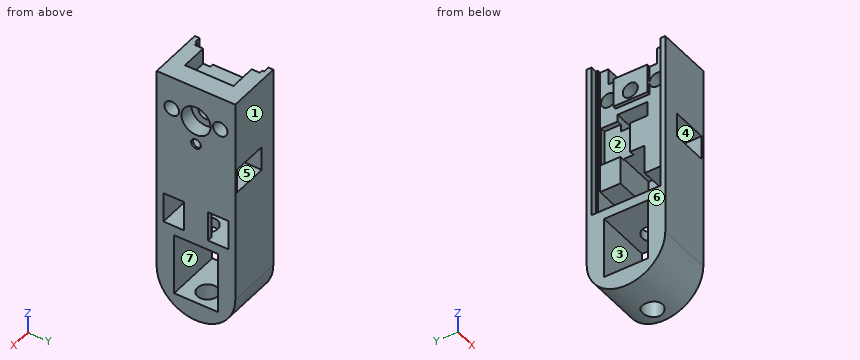
```python
from build123d import *

# Parameters (mm, degrees)
SKETCH_W         = 4.2
SKETCH_H         = 6.2
EXTRUDE_DEPTH    = 11.5
SKETCH001_W      = 14.2
SKETCH001_H      = 32.3
SKETCH001_R      = 1.55
EXTRUDE001_DEPTH = 1.3
SKETCH003_W      = 10
SKETCH003_H      = 4.382065
EXTRUDE003_DEPTH = 7.5
SKETCH004_W      = 13.4
SKETCH004_H      = 32.3
SKETCH004_W_2    = 7
SKETCH004_H_2    = 6
EXTRUDE004_DEPTH = 2
SKETCH005_W      = 6
SKETCH005_H      = 8
EXTRUDE005_DEPTH = 3
SKETCH009_W      = 18
SKETCH009_H      = 5
EXTRUDE013_DEPTH = 7.5
SKETCH012_W      = 9
SKETCH012_H      = 12.7
EXTRUDE014_DEPTH = 11.5
SKETCH011_R      = 2.08
EXTRUDE012_DEPTH = 20
SKETCH002_W      = 5
SKETCH002_H      = 12.2
EXTRUDE011_DEPTH = 10.5
EXTRUDE015_DEPTH = 3
SKETCH014_R      = 1
EXTRUDE016_DEPTH = 12
SKETCH015_R      = 1.5
EXTRUDE017_DEPTH = 11.5
SKETCH016_R      = 3
EXTRUDE018_DEPTH = 3
SKETCH010_R      = 1.55
EXTRUDE010_DEPTH = 12
EXTRUDE006_DEPTH = 11.5


with BuildPart() as extrude_body:
    # Sketch → Extrude (new body)
    with BuildSketch(Plane.YZ):
        with Locations((4.6, 3.1)):
            Rectangle(SKETCH_W, SKETCH_H)
    extrude(amount=EXTRUDE_DEPTH)


with BuildPart() as extrude001:
    # Sketch001 → Extrude001 (new body)
    with BuildSketch(Plane.YZ):
        with Locations((0, 16.15)):
            Rectangle(SKETCH001_W, SKETCH001_H)
        with Locations((0, 25)):
            Circle(SKETCH001_R, mode=Mode.SUBTRACT)
    extrude(amount=EXTRUDE001_DEPTH)


with BuildPart() as extrude003:
    # Sketch003 → Extrude003 (new body)
    with BuildSketch(Plane.YZ):
        with Locations((0, 31.191032)):
            Rectangle(SKETCH003_W, SKETCH003_H)
    extrude(amount=EXTRUDE003_DEPTH)


with BuildPart() as extrude004:
    # Sketch004 → Extrude004 (new body)
    with BuildSketch(Plane.YZ):
        with Locations((0, 16.15)):
            Rectangle(SKETCH004_W, SKETCH004_H)
        with Locations((0, 26)):
            Rectangle(SKETCH004_W_2, SKETCH004_H_2, mode=Mode.SUBTRACT)
    extrude(amount=EXTRUDE004_DEPTH)


with BuildPart() as extrude005:
    # Sketch005 → Extrude005 (new body)
    with BuildSketch(Plane.YZ):
        with Locations((3.5, 16)):
            Rectangle(SKETCH005_W, SKETCH005_H)
    extrude(amount=EXTRUDE005_DEPTH)


with BuildPart() as board:
    # Part__Mirroring: instance of Extrude body
    add(extrude_body.part.mirror(Plane(origin=(0, 0, 0), x_dir=(1, 0, 0), z_dir=(0, 1, 0))))

    # Fusion: union Extrude body, Extrude001, Extrude003, Extrude004, Extrude005
    add(extrude_body.part)
    add(extrude001.part)
    add(extrude003.part)
    add(extrude004.part)
    add(extrude005.part)


with BuildPart() as obj1:
    # Sketch009 → Extrude013 (new body)
    with BuildSketch(Plane.YZ):
        with Locations((0, 15.2)):
            Rectangle(SKETCH009_W, SKETCH009_H)
    extrude(amount=EXTRUDE013_DEPTH)


with BuildPart() as obj1_1:
    # Extrude013 placement: moved
    add(obj1.part.moved(Location((3.5, 0, 0))))


with BuildPart() as obj2:
    # Sketch012 → Extrude014 (new body)
    with BuildSketch(Plane.YZ):
        with Locations((0, -8.35)):
            Rectangle(SKETCH012_W, SKETCH012_H)
    extrude(amount=EXTRUDE014_DEPTH)


with BuildPart() as percageaxe:
    # Sketch011 → Extrude012 (new body)
    with BuildSketch(Plane.XY):
        with Locations((8, 0)):
            Circle(SKETCH011_R)
    extrude(amount=-EXTRUDE012_DEPTH)


with BuildPart() as obj3:
    # Sketch002 → Extrude011 (new body)
    with BuildSketch(Plane.YZ):
        with Locations((0, 6.1)):
            Rectangle(SKETCH002_W, SKETCH002_H)
    extrude(amount=EXTRUDE011_DEPTH)


with BuildPart() as obj4:
    # Sketch013 → Extrude015 (new body)
    with BuildSketch(Plane.XY):
        with BuildLine():
            ThreePointArc((6.780369, -2.85), (11.1, 0), (6.780369, 2.85))
            ThreePointArc((6.780369, 2.85), (6.183233, 3.036857), (5.560738, 3.1))
            Line((5.560738, 3.1), (0, 3.1))
            Line((0, -3.1), (0, 3.1))
            Line((5.560738, -3.1), (0, -3.1))
            ThreePointArc((5.560738, -3.1), (6.183233, -3.036857), (6.780369, -2.85))
        make_face()
    extrude(amount=EXTRUDE015_DEPTH)


with BuildPart() as obj4_1:
    # Extrude015 placement: moved
    add(obj4.part.moved(Location((0, 0, 18.5))))


with BuildPart() as obj5:
    # Sketch014 → Extrude016 (new body)
    with BuildSketch(Plane.YZ):
        Circle(SKETCH014_R)
    extrude(amount=EXTRUDE016_DEPTH)


with BuildPart() as obj5_1:
    # Extrude016 placement: moved
    add(obj5.part.moved(Location((0, 0, 20))))


with BuildPart() as obj6:
    # Sketch015 → Extrude017 (new body)
    with BuildSketch(Plane.YZ):
        with Locations((-5, 25.5)):
            Circle(SKETCH015_R)
        with Locations((5, 25.5)):
            Circle(SKETCH015_R)
    extrude(amount=EXTRUDE017_DEPTH)


with BuildPart() as obj7:
    # Sketch016 → Extrude018 (new body)
    with BuildSketch(Plane.YZ):
        with Locations((0, 25)):
            Circle(SKETCH016_R)
    extrude(amount=EXTRUDE018_DEPTH)


with BuildPart() as obj7_1:
    # Extrude018 placement: moved
    add(obj7.part.moved(Location((8.5, 0, 0))))


with BuildPart() as fusion002:
    # Sketch010 → Extrude010 (new body)
    with BuildSketch(Plane.YZ):
        with Locations((0, 25)):
            Circle(SKETCH010_R)
    extrude(amount=EXTRUDE010_DEPTH)

    # Fusion002: union obj1, obj2, PercageAxe, obj3, obj4, obj5, obj6, obj7
    add(obj1_1.part)
    add(obj2.part)
    add(percageaxe.part)
    add(obj3.part)
    add(obj4_1.part)
    add(obj5_1.part)
    add(obj6.part)
    add(obj7_1.part)


with BuildPart() as cut001:
    # Sketch006 → Extrude006 (new body)
    with BuildSketch(Plane.YZ):
        with BuildLine():
            Line((-8.1, 32.3), (8.1, 32.3))
            Line((8.1, -10.5), (8.1, 32.3))
            ThreePointArc((-8.1, -10.5), (0, -18.6), (8.1, -10.5))
            Line((-8.1, 32.3), (-8.1, -10.5))
        make_face()
    extrude(amount=EXTRUDE006_DEPTH)

    # Cut: cut Fusion002
    add(fusion002.part, mode=Mode.SUBTRACT)

    # Cut001: cut Board
    add(board.part, mode=Mode.SUBTRACT)


solid = cut001.part
```
Work out the finished part from the listing and answer in its coordinate system (mm). Face numbers are marked on the shaded views. A direction names the side the tool comes from. Round coordinates to 2 decimals unless told otherwise and drop trailing zeros. Loops run counter-clockwise (first coordinate to the right, second up) from the corner with the lowest first, then second, coordinate; pieces in that order, holes last. Notation, with made-up numbers: (5, 58.5) -> (34, 58.5) arc R16 ccw to (34, 79.5) -> close; hole circle Ø10 at (26, 9). An arc over 180 degrees is marked (long way). Write each question's results on one line, items separated by ' | '. Start each with the question number.
1. Section B-B (y = 0) is taken. State how many separate pieces and enclosed holes the cut face has, plus the area to 3 significant figures.
2. Find the intervals of material crossed by probe 1 along X at (y, z) = (2, 17.5); probe 2 along Z at (x, y) = (9.5, -5); probe 3 along Y at (x, z) = (9.5, 2.5), in increasing order. Write a range as from..to.
3. A tool of negligible diameter and unlimited length cuts with its end or side. For the marked faces 1, 2 and 3, from which of +Z, -Z, +X, -X, +Y, -Y can it reach the whole face along a straight path? Write none if from no direction.
4. For a pull along X with two mould halves and no side action, classify the marked faces 4, 5, 6 and 7 as +X half, -X half, draft (parallel to the pull), parting line (faces both ways), or undercut.
5. Section A-A (z = -3) is taken. Determine the outline of the cut face in (x, y).
6. Given pin 1 Ø2 at (x, y) = (9.5, 3.5) entering from -Z; pin 2 Ø6.5 at (y, z) = (1.5, 26.5) entering from -X; pin 3 Ø1 at (y, z) = (2.5, -9) entering from -X; pin 4 Ø3.5 at (x, y) = (8, 0) entering from -Z, each flat-ended and moving along its own axis, determine where each tip first touches the part or whether it passes through.
Evaluation:
1) separate pieces: 6 | enclosed holes: 1 | area: 127 mm2
2) probe 1: x = 3..3.5, 11..11.5 | probe 2: z = -16.87..0, 6.2..12.7, 17.7..24, 27..32.3 | probe 3: y = -8.1..-6.7, 6.7..8.1
3) face 1: +Z, -Z, +X, -X, +Y | face 2: -X | face 3: +X, -X
4) face 4: undercut | face 5: undercut | face 6: -X half | face 7: draft
5) outline: (0, -8.1) -> (11.5, -8.1) -> (11.5, -4.5) -> (0, -4.5) -> close; (0, 4.5) -> (11.5, 4.5) -> (11.5, 8.1) -> (0, 8.1) -> close
6) pin 1: stops at z = -18.2 | pin 2: stops at x = 1.3 | pin 3: passes through | pin 4: stops at z = 12.2
